Build history of the part. All positions in model axes, mm. Face numbers are marked on the shaded views. A direction names the side the tool comes from. Give positions to 0.01 mm unless a question says otherwise; leave off trailing zeros. Order: outer loops, then holes, each group sorted by start corner. A loop starts at its lowest first (then second) coordinate and runs counter-clockwise, first axis right, second up. Notation, with made-up numbers: (-11, 36.5) -> (27, 36.5) arc R21 ccw to (27, 47.5) -> close; hole circle Ø7 at (-26.5, 0.25). An arc over 180 degrees is marked (long way). Write item = value, one per line. Start each with the question number.
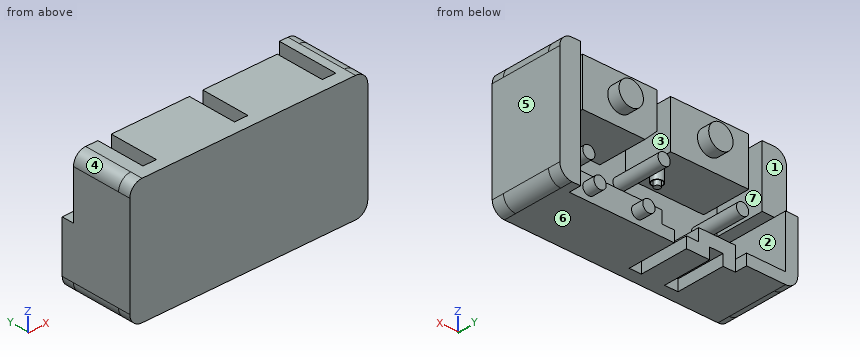
from build123d import *

# Parameters (mm, degrees)
SZKIC1_W                     = 19.5
SZKIC1_H                     = 10.2
DODANIE_WYCI_GNI_CIE2_DEPTH  = 1
ZAOKR_GLENIE1_R              = 1
ZAOKR_GLENIE2_R              = 1
ZAOKR_GLENIE3_R              = 1
ZAOKR_GLENIE4_R              = 1
SZKIC4_R                     = 0.5
SZKIC4_W                     = 6.4
SZKIC4_H                     = 3.9
DODANIE_WYCI_GNI_CIE4_DEPTH  = 4
ZAOKR_GLENIE5_R              = 1
ZAOKR_GLENIE6_R              = 1
ZAOKR_GLENIE7_R              = 1
ZAOKR_GLENIE8_R              = 1
SZKIC8_R                     = 1
SZKIC8_R_2                   = 0.5
SZKIC8_W                     = 1.7
SZKIC8_H                     = 10.2
DODANIE_WYCI_GNI_CIE12_DEPTH = 1
ZAOKR_GLENIE12_R             = 1
SZKIC12_R                    = 0.25
DODANIE_WYCI_GNI_CIE14_DEPTH = 1.3
SZKIC15_R                    = 0.450396943
SZKIC15_R_2                  = 0.398132247
DODANIE_WYCI_GNI_CIE15_DEPTH = 1


with BuildPart() as part:
    # Szkic1 → Dodanie-wyciągnięcie2 (new body)
    with BuildSketch(Plane(origin=(0, 0, 0), x_dir=(1, 0, 0), z_dir=(0, 1, 0))):
        Rectangle(SZKIC1_W, SZKIC1_H)
    extrude(amount=DODANIE_WYCI_GNI_CIE2_DEPTH)

    # Zaokrąglenie1
    zaokr_glenie1_edges = [part.edges().sort_by_distance(p)[0] for p in [
        (-9.75, 0.5, 5.1),
    ]]
    fillet(zaokr_glenie1_edges, radius=ZAOKR_GLENIE1_R)

    # Zaokrąglenie2
    zaokr_glenie2_edges = [part.edges().sort_by_distance(p)[0] for p in [
        (-9.75, 0.5, -5.1),
    ]]
    fillet(zaokr_glenie2_edges, radius=ZAOKR_GLENIE2_R)

    # Zaokrąglenie3
    zaokr_glenie3_edges = [part.edges().sort_by_distance(p)[0] for p in [
        (9.75, 0.5, 5.1),
    ]]
    fillet(zaokr_glenie3_edges, radius=ZAOKR_GLENIE3_R)

    # Zaokrąglenie4
    zaokr_glenie4_edges = [part.edges().sort_by_distance(p)[0] for p in [
        (9.75, 0.5, -5.1),
    ]]
    fillet(zaokr_glenie4_edges, radius=ZAOKR_GLENIE4_R)

    # Szkic4 → Dodanie-wyciągnięcie4 (add)
    with BuildSketch(Plane(origin=(0, 1, 0), x_dir=(1, 0, 0), z_dir=(0, 1, 0))):
        with Locations(Location((0.279656429, -0.460729366, 0), (0, 0, 270))):
            Circle(SZKIC4_R)
        with Locations(Location((-6.15, 0.4, 0), (0, 0, 270))):
            Circle(SZKIC4_R)
        with Locations(Location((6.45, 1.595263288, 0), (0, 0, 270))):
            Circle(SZKIC4_R)
        Polygon((-8.75, -0.1), (-7.75, -0.1), (-7.75, -5.1), (-9.75, -5.1), (-9.75, 5.1), (-4.55, 5.1), (-4.55, 4.195263288), (-3.45, 4.195263288), (-3.45, 5.1), (-1.552474018, 5.1), (-1.552474018, 4.195263288), (-2.55, 4.195263288), (-2.55, 3.195263288), (-5.55, 3.195263288), (-5.55, 4.195263288), (-8.75, 4.195263288), align=None)
        with Locations((-3.45, -3.15)):
            Rectangle(SZKIC4_W, SZKIC4_H)
        Polygon((0.85, -5.1), (6.95, -5.1), (6.95, -1.2), (1.85, -1.2), (0.85, -2.2), align=None)
        Polygon((8.05, -5.1), (9.75, -5.1), (9.75, 5.1), (-0.553774682, 5.1), (-0.553774682, 4.195263288), (0.45, 4.195263288), (0.45, 3.195263288), (8.05, 3.195263288), align=None)
    extrude(amount=DODANIE_WYCI_GNI_CIE4_DEPTH)

    # Zaokrąglenie5
    zaokr_glenie5_edges = [part.edges().sort_by_distance(p)[0] for p in [
        (-9.75, 3, 5.1),
    ]]
    fillet(zaokr_glenie5_edges, radius=ZAOKR_GLENIE5_R)

    # Zaokrąglenie6
    zaokr_glenie6_edges = [part.edges().sort_by_distance(p)[0] for p in [
        (-9.75, 3, -5.1),
    ]]
    fillet(zaokr_glenie6_edges, radius=ZAOKR_GLENIE6_R)

    # Zaokrąglenie7
    zaokr_glenie7_edges = [part.edges().sort_by_distance(p)[0] for p in [
        (9.75, 3, -5.1),
    ]]
    fillet(zaokr_glenie7_edges, radius=ZAOKR_GLENIE7_R)

    # Zaokrąglenie8
    zaokr_glenie8_edges = [part.edges().sort_by_distance(p)[0] for p in [
        (9.75, 3, 5.1),
    ]]
    fillet(zaokr_glenie8_edges, radius=ZAOKR_GLENIE8_R)

    # Szkic8 → Dodanie-wyciągnięcie12 (add)
    with BuildSketch(Plane(origin=(0, 5, 0), x_dir=(1, 0, 0), z_dir=(0, 1, 0))):
        with Locations(Location((-3.45, -3.15, 0), (0, 0, 90))):
            Circle(SZKIC8_R)
        with Locations(Location((3.9, -3.15, 0), (0, 0, 90))):
            Circle(SZKIC8_R)
        with Locations(Location((6.45, 4.195263288, 0), (0, 0, 90))):
            Circle(SZKIC8_R_2)
        with Locations(Location((2.45, 4.195263288, 0), (0, 0, 90))):
            Circle(SZKIC8_R_2)
        Polygon((-8.75, -0.1), (-9.75, -0.1), (-9.75, 5.1), (-5.55, 5.1), (-5.55, 4.195263288), (-8.75, 4.195263288), align=None)
        with Locations((8.9, 0)):
            Rectangle(SZKIC8_W, SZKIC8_H)
    extrude(amount=DODANIE_WYCI_GNI_CIE12_DEPTH)

    # Zaokrąglenie12
    zaokr_glenie12_edges = [part.edges().sort_by_distance(p)[0] for p in [
        (9.75, 5.5, -5.1),
        (9.75, 5.5, 5.1),
        (-9.75, 5.5, -5.1),
    ]]
    fillet(zaokr_glenie12_edges, radius=ZAOKR_GLENIE12_R - 0.0001)  # a hair under: the kernel refuses the full size

    # Szkic12 → Dodanie-wyciągnięcie14 (add)
    with BuildSketch(Plane(origin=(0, 0, 1.2), x_dir=(-1, 0, 0), z_dir=(0, 0, -1))):
        with Locations(Location((1, 3, 0), (0, 0, 180))):
            Circle(SZKIC12_R)
    extrude(amount=DODANIE_WYCI_GNI_CIE14_DEPTH)

    # Szkic15 → Dodanie-wyciągnięcie15 (add)
    with BuildSketch(Plane(origin=(0, 0, 1.2), x_dir=(-1, 0, 0), z_dir=(0, 0, -1))):
        with Locations(Location((1, 3, 0), (0, 0, 180))):
            Circle(SZKIC15_R)
        with Locations((1, 3)):
            Circle(SZKIC15_R_2, mode=Mode.SUBTRACT)
    extrude(amount=DODANIE_WYCI_GNI_CIE15_DEPTH)


solid = part.part
(1) Flat gauge pin, fed straight in: P1, Ø0.8, axis at x = -6.5, z = -0.5, coming from the +Y side. Where does the tip first touch, or does it go through?
(2) Cut at A-A, the plane y = 5.25. Give the cut face in (x, z), plus the area to 3 significant figures.
(3) 3-axis set-ups, long thin cutter, end or side, ignore diameter. For the marked faces 1, 2 and 3: which of +Z, -Z, +X, -X, +Y, -Y reach the whole face in a straight line?
(4) Mould opens along X. For the marked faces 4, 5, 6 and 7 say: released by +X, released by -X, zero draft, split by the parting line, or undercut.
(5) Cut at B-B, the plane x = -6.15. Give the cut face in (y, z), plus the area to 3 significant figures.
(6) Cut at C-C, the plane z = 3.15. Give the cut face in (x, y), plus the area to 3 significant figures.
(7) Wall check: line 1 (X direction, y = 1.1, z = 0.5); line 2 (X direction, y = 3.15, z = 3.75); line 3 (Z direction, x = -2, y = 4.2). Give the ranges that are in metal, low to high. Write a range as [from, to].
(8) Cut at D-D, the plane x = 1.25. Give the cut face in (y, z).
Results:
q1.P1 = 5
q2.outline = (-9.75, -4.1) arc R1 ccw to (-8.75, -5.1) -> (-5.55, -5.1) -> (-5.55, -4.2) -> (-8.75, -4.2) -> (-8.75, 0.1) -> (-9.75, 0.1) -> close; circle Ø2 at (-3.45, 3.15); circle Ø1 at (2.45, -4.2); circle Ø2 at (3.9, 3.15); circle Ø1 at (6.45, -4.2); (8.05, -5.1) -> (8.75, -5.1) arc R1 ccw to (9.75, -4.1) -> (9.75, 4.1) arc R1 ccw to (8.75, 5.1) -> (8.05, 5.1) -> close
q2.area = 32.6 mm2
q3.face_1 = +Z, -X, +Y
q3.face_2 = +Y
q3.face_3 = +Z, +Y
q4.face_4 = released by -X
q4.face_5 = released by +X
q4.face_6 = zero draft
q4.face_7 = undercut
q5.outline = (0, -5.1) -> (6, -5.1) -> (6, -4.2) -> (1, -4.2) -> (1, -0.9) -> (5, -0.9) -> (5, 0.1) -> (1, 0.1) -> (1, 1.2) -> (5, 1.2) -> (5, 5.1) -> (0, 5.1) -> close
q5.area = 34.3 mm2
q6.outline = (-9.75, 0) -> (9.75, 0) -> (9.75, 6) -> (8.05, 6) -> (8.05, 1) -> (6.95, 1) -> (6.95, 5) -> (4.9, 5) -> (4.9, 6) -> (2.9, 6) -> (2.9, 5) -> (0.85, 5) -> (0.85, 1) -> (-0.25, 1) -> (-0.25, 5) -> (-2.45, 5) -> (-2.45, 6) -> (-4.45, 6) -> (-4.45, 5) -> (-6.65, 5) -> (-6.65, 1) -> (-7.75, 1) -> (-7.75, 5) -> (-9.75, 5) -> close
q6.area = 90.0 mm2
q7.line_1 = [-9.75, -7.75], [-0.22, 0.78], [8.05, 9.75]
q7.line_2 = [-9.75, -7.75], [-6.65, -0.25], [0.85, 6.95], [8.05, 9.75]
q7.line_3 = [-5.1, -4.2], [1.2, 5.1]
q8.outline = (0, -5.1) -> (5, -5.1) -> (5, -3.2) -> (1, -3.2) -> (1, 1.8) -> (5, 1.8) -> (5, 5.1) -> (0, 5.1) -> close
